```python
from build123d import *

# Parameters (mm, degrees)
F1_DEPTH = 5


with BuildPart() as f1:
    # F0 (on Right) → F1 (new body)
    with BuildSketch(Plane.YZ):
        Polygon((104.411765, 40.84024), (110.185267, 40.84024), (110.185267, 45.84024), (-101.361738, 45.84024), (-101.361738, 40.84024), (-95.588235, 40.84024), (-89.814733, 40.84024), (-48.314733, 40.84024), (-42.861738, 40.84024), (-1.361738, 40.84024), (4.411765, 40.84024), (10.185267, 40.84024), (51.685267, 40.84024), (57.138262, 40.84024), (98.638262, 40.84024), align=None)
        Polygon((-89.814733, 40.84024), (-95.588235, 40.84024), (-92.861738, 36.117808), (-51.361738, -35.7623), (-45.588235, -35.7623), (-48.314733, -31.039869), align=None)
        Polygon((-98.314733, 36.117808), (-98.314733, -35.7623), (-92.861738, -35.7623), (-92.861738, 36.117808), (-95.588235, 40.84024), align=None)
        Polygon((-48.314733, 40.84024), (-48.314733, -31.039869), (-45.588235, -35.7623), (-42.861738, -31.039869), (-42.861738, 40.84024), align=None)
        Polygon((-42.861738, -31.039869), (-45.588235, -35.7623), (-39.814733, -35.7623), (1.685267, 36.117808), (4.411765, 40.84024), (-1.361738, 40.84024), align=None)
        Polygon((-101.361738, 40.84024), (-145.588235, -35.7623), (-139.814733, -35.7623), (-98.314733, 36.117808), (-95.588235, 40.84024), align=None)
        Polygon((-145.588235, -41.7623), (154.411765, -41.7623), (154.411765, -35.7623), (148.638262, -35.7623), (107.138262, -35.7623), (101.685267, -35.7623), (60.185267, -35.7623), (54.411765, -35.7623), (48.638262, -35.7623), (7.138262, -35.7623), (1.685267, -35.7623), (-39.814733, -35.7623), (-45.588235, -35.7623), (-51.361738, -35.7623), (-92.861738, -35.7623), (-98.314733, -35.7623), (-139.814733, -35.7623), (-145.588235, -35.7623), align=None)
        Polygon((1.685267, -35.7623), (7.138262, -35.7623), (7.138262, 36.117808), (4.411765, 40.84024), (1.685267, 36.117808), align=None)
        Polygon((48.638262, -35.7623), (54.411765, -35.7623), (51.685267, -31.039869), (10.185267, 40.84024), (4.411765, 40.84024), (7.138262, 36.117808), align=None)
        Polygon((54.411765, -35.7623), (57.138262, -31.039869), (57.138262, 40.84024), (51.685267, 40.84024), (51.685267, -31.039869), align=None)
        Polygon((101.685267, 36.117808), (104.411765, 40.84024), (98.638262, 40.84024), (57.138262, -31.039869), (54.411765, -35.7623), (60.185267, -35.7623), align=None)
        Polygon((101.685267, -35.7623), (107.138262, -35.7623), (107.138262, 36.117808), (104.411765, 40.84024), (101.685267, 36.117808), align=None)
        Polygon((148.638262, -35.7623), (154.411765, -35.7623), (110.185267, 40.84024), (104.411765, 40.84024), (107.138262, 36.117808), align=None)
    extrude(amount=F1_DEPTH)


solid = f1.part
```
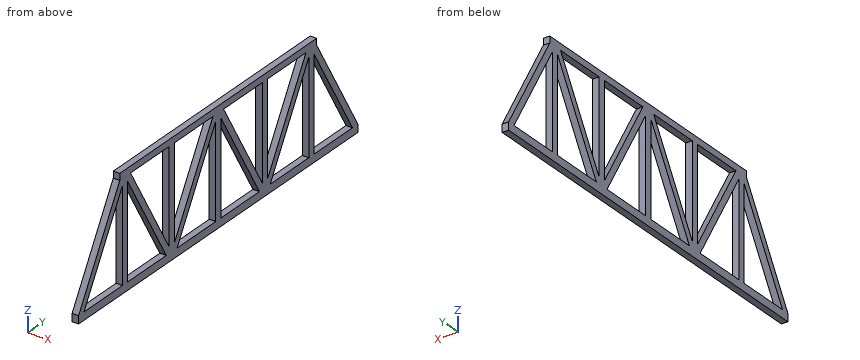
Here's how the part is built. I have some questions about the finished solid (model axes, mm). Give positions to 0.01 mm unless a question says otherwise; leave off trailing zeros. Order: outer loops, then holes, each group sorted by start corner. A loop starts at its lowest first (then second) coordinate and runs counter-clockwise, first axis right, second up. Notation, with made-up numbers: (10, 9.25) -> (56, 9.25) arc R33 ccw to (56, 42.25) -> close; hole circle Ø3 at (55.5, 84). An arc over 180 degrees is marked (long way). Use CSV: the item, a comma, the result in double quotes. Start each with the question number.
Item 1: I'm going to push flat-ended pins straight in: P1, Ø2.5, axis at x = 3.5, z = 13, coming from the +Y side; P2, Ø3, axis at x = 1, z = 17.5, coming from the -Y side; P3, Ø1.5, axis at x = 3, z = 30, coming from the -Y side. Where does each tip first touch, or does it pass through?
Item 2: Suppose I cut it at B-B (y = 79.5). List the corners of the cut face in (x, z) for me, and give its area (3 significant figures).
Item 3: Suppose I cut it at A-A (y = -122). List the corners of the cut face in (x, z) for me.
Item 4: Suppose I cut it at C-C (x = 3.95). Give the number of separate pieces and of enclosed holes in the cut face, and give its area (3 significant figures).
Item 5: If I drill on probe 1 along Z at (x, y) = (4.4, 25); probe 2 along Z at (x, y) = (1.15, -15.5); probe 3 along Z at (x, y) = (2.95, 59), over which ranges is the centre line in solid material (lowest first)? Write a range as [from, to].
Answer block:
1,P1,"stops at y = 126.98"
1,P2,"stops at y = -115.7"
1,P3,"stops at y = -108.05"
2,outline,"(0, -41.76) -> (5, -41.76) -> (5, -35.76) -> (0, -35.76) -> close; (0, -2.31) -> (5, -2.31) -> (5, 7.69) -> (0, 7.69) -> close; (0, 40.84) -> (5, 40.84) -> (5, 45.84) -> (0, 45.84) -> close"
2,area,"105 mm^2"
3,outline,"(0, -41.76) -> (5, -41.76) -> (5, -35.76) -> (0, -35.76) -> close; (0, -4.91) -> (5, -4.91) -> (5, 5.09) -> (0, 5.09) -> close"
4,separate pieces,"1"
4,enclosed holes,"10"
4,area,"7,540 mm^2"
5,probe 1,"z = [-41.76, -35.76], [5.18, 15.18], [40.84, 45.84]"
5,probe 2,"z = [-41.76, -35.76], [6.35, 16.35], [40.84, 45.84]"
5,probe 3,"z = [-41.76, -27.82], [40.84, 45.84]"
